```python
from build123d import *

# Parameters (mm, degrees)
BOSS_EXTRUDE1_DEPTH = 6.35
SKETCH3_R           = 3.96875
CUT_EXTRUDE1_DEPTH  = 7.35
SKETCH5_W           = 6.35
SKETCH5_H           = 12.7
CUT_EXTRUDE3_DEPTH  = 7.35
LPATTERN1_COUNT     = 16
LPATTERN1_PITCH     = 25.4
SKETCH6_W           = 6.35
SKETCH6_H           = 12.7
CUT_EXTRUDE4_DEPTH  = 7.35
LPATTERN2_COUNT     = 11
LPATTERN2_PITCH     = 25.4
SKETCH7_W           = 6.35
SKETCH7_H           = 12.7
SKETCH7_W_2         = 12.7
SKETCH7_H_2         = 6.35
CUT_EXTRUDE5_DEPTH  = 7.35
CUT_EXTRUDE6_DEPTH  = 7.35
LPATTERN3_COUNT     = 10
LPATTERN3_PITCH     = 25.4
SKETCH9_W           = 12.7
SKETCH9_H           = 6.35
CUT_EXTRUDE7_DEPTH  = 7.35
LPATTERN4_COUNT     = 8
LPATTERN4_PITCH     = 25.4
SKETCH10_R          = 3.175
CUT_EXTRUDE8_DEPTH  = 7.35
SKETCH11_R          = 3.96875
CUT_EXTRUDE9_DEPTH  = 7.35
SKETCH12_W          = 6.35
SKETCH12_H          = 12.7
CUT_EXTRUDE13_DEPTH = 7.35
CUT_EXTRUDE15_DEPTH = 7.35
CUT_EXTRUDE16_DEPTH = 7.35
SKETCH17_W          = 12.7
SKETCH17_H          = 6.35
CUT_EXTRUDE17_DEPTH = 7.35
LPATTERN5_COUNT     = 17
LPATTERN5_PITCH     = 25.4
LPATTERN6_COUNT     = 2
LPATTERN6_PITCH     = 120.65
SKETCH18_W          = 12.7
SKETCH18_H          = 6.35
CUT_EXTRUDE18_DEPTH = 7.35
LPATTERN7_COUNT     = 5
LPATTERN7_PITCH     = 25.4
CUT_EXTRUDE19_DEPTH = 7.35
SKETCH20_W          = 101.6
SKETCH20_H          = 57.15
CUT_EXTRUDE20_DEPTH = 7.35
CUT_EXTRUDE21_DEPTH = 7.35
CUT_EXTRUDE22_DEPTH = 7.35
BOSS_EXTRUDE4_DEPTH = 6.35
BOSS_EXTRUDE5_DEPTH = 6.35
SKETCH29_R          = 2.54
CUT_EXTRUDE23_DEPTH = 7.35
SKETCH30_R          = 1.75
CUT_EXTRUDE24_DEPTH = 7.35
SKETCH31_R          = 1.75
CUT_EXTRUDE25_DEPTH = 7.35
FILLET2_R           = 6.35


with BuildPart() as part:
    # Sketch2 → Boss-Extrude1 (new body)
    with BuildSketch(Plane(origin=(0, 0, 0), x_dir=(0, 0, -1), z_dir=(1, 0, 0))):
        Polygon((0, 0), (0, 294.450076882), (215.9, 419.1), (431.8, 419.1), (431.8, 0), (241.3, 0), (241.3, 38.1), (127, 38.1), (127, 0), align=None)
    extrude(amount=BOSS_EXTRUDE1_DEPTH)

    # Sketch3 → Cut-Extrude1 (cut, through all)
    with BuildSketch(Plane(origin=(6.35, 0, 0), x_dir=(0, 0, -1), z_dir=(1, 0, 0))):
        with Locations((63.5, 38.1)):
            Circle(SKETCH3_R)
        with Locations((368.3, 38.1)):
            Circle(SKETCH3_R)
    extrude(amount=-CUT_EXTRUDE1_DEPTH, mode=Mode.SUBTRACT)

    # Sketch5 → Cut-Extrude3 (cut, through all)
    with BuildSketch(Plane(origin=(6.35, 0, 0), x_dir=(0, 0, -1), z_dir=(1, 0, 0))):
        with Locations((428.625, 19.05)):
            Rectangle(SKETCH5_W, SKETCH5_H)
    cut_extrude3 = extrude(amount=-CUT_EXTRUDE3_DEPTH, mode=Mode.SUBTRACT)

    # LPattern1: Cut-Extrude3 ×16
    with Locations(*[(0, i * LPATTERN1_PITCH, 0) for i in range(1, LPATTERN1_COUNT)]):
        add(cut_extrude3, mode=Mode.SUBTRACT)

    # Sketch6 → Cut-Extrude4 (cut, through all)
    with BuildSketch(Plane(origin=(6.35, 0, 0), x_dir=(0, 0, -1), z_dir=(1, 0, 0))):
        with Locations((3.175, 19.05)):
            Rectangle(SKETCH6_W, SKETCH6_H)
    cut_extrude4 = extrude(amount=-CUT_EXTRUDE4_DEPTH, mode=Mode.SUBTRACT)

    # LPattern2: Cut-Extrude4 ×11
    with Locations(*[(0, i * LPATTERN2_PITCH, 0) for i in range(1, LPATTERN2_COUNT)]):
        add(cut_extrude4, mode=Mode.SUBTRACT)

    # Sketch7 → Cut-Extrude5 (cut, through all)
    with BuildSketch(Plane(origin=(6.35, 0, 0), x_dir=(0, 0, -1), z_dir=(1, 0, 0))):
        with Locations((123.825, 19.05)):
            Rectangle(SKETCH7_W, SKETCH7_H)
        with Locations((133.35, 41.275)):
            Rectangle(SKETCH7_W_2, SKETCH7_H_2)
        with Locations((158.75, 41.275)):
            Rectangle(SKETCH7_W_2, SKETCH7_H_2)
        with Locations((184.15, 41.275)):
            Rectangle(SKETCH7_W_2, SKETCH7_H_2)
        with Locations((244.475, 19.05)):
            Rectangle(SKETCH7_W, SKETCH7_H)
        with Locations((209.55, 41.275)):
            Rectangle(SKETCH7_W_2, SKETCH7_H_2)
        with Locations((234.95, 41.275)):
            Rectangle(SKETCH7_W_2, SKETCH7_H_2)
    extrude(amount=-CUT_EXTRUDE5_DEPTH, mode=Mode.SUBTRACT)

    # Sketch8 → Cut-Extrude6 (cut, through all)
    with BuildSketch(Plane(origin=(6.35, 0, 0), x_dir=(0, 0, -1), z_dir=(1, 0, 0))):
        Polygon((201.93507044, 411.037344159), (212.933593068, 417.387344159), (216.108593068, 411.888082845), (205.11007044, 405.538082845), align=None)
    cut_extrude6 = extrude(amount=-CUT_EXTRUDE6_DEPTH, mode=Mode.SUBTRACT)

    # LPattern3: Cut-Extrude6 ×10
    with Locations(*[Vector(0, -0.5, 0.866025404) * (i * LPATTERN3_PITCH) for i in range(1, LPATTERN3_COUNT)]):
        add(cut_extrude6, mode=Mode.SUBTRACT)

    # Sketch9 → Cut-Extrude7 (cut, through all)
    with BuildSketch(Plane(origin=(6.35, 0, 0), x_dir=(0, 0, -1), z_dir=(1, 0, 0))):
        with Locations((412.75, 415.925)):
            Rectangle(SKETCH9_W, SKETCH9_H)
    cut_extrude7 = extrude(amount=-CUT_EXTRUDE7_DEPTH, mode=Mode.SUBTRACT)

    # LPattern4: Cut-Extrude7 ×8
    with Locations(*[(0, 0, i * LPATTERN4_PITCH) for i in range(1, LPATTERN4_COUNT)]):
        add(cut_extrude7, mode=Mode.SUBTRACT)

    # Sketch10 → Cut-Extrude8 (cut, through all)
    with BuildSketch(Plane(origin=(6.35, 0, 0), x_dir=(0, 0, -1), z_dir=(1, 0, 0))):
        with Locations((222.25, 273.05)):
            Circle(SKETCH10_R)
        with Locations((222.25, 57.15)):
            Circle(SKETCH10_R)
        with Locations((146.05, 57.15)):
            Circle(SKETCH10_R)
        with Locations((146.05, 273.05)):
            Circle(SKETCH10_R)
    extrude(amount=-CUT_EXTRUDE8_DEPTH, mode=Mode.SUBTRACT)

    # Sketch11 → Cut-Extrude9 (cut, through all)
    with BuildSketch(Plane(origin=(6.35, 0, 0), x_dir=(0, 0, -1), z_dir=(1, 0, 0))):
        with Locations((38.1, 260.35)):
            Circle(SKETCH11_R)
        with Locations((266.7, 260.35)):
            Circle(SKETCH11_R)
    extrude(amount=-CUT_EXTRUDE9_DEPTH, mode=Mode.SUBTRACT)

    # Sketch12 → Cut-Extrude13 (cut, through all)
    with BuildSketch(Plane(origin=(6.35, 0, 0), x_dir=(0, 0, -1), z_dir=(1, 0, 0))):
        with Locations((123.825, 44.45)):
            Rectangle(SKETCH12_W, SKETCH12_H)
        with Locations((123.825, 69.85)):
            Rectangle(SKETCH12_W, SKETCH12_H)
        with Locations((123.825, 95.25)):
            Rectangle(SKETCH12_W, SKETCH12_H)
        with Locations((123.825, 120.65)):
            Rectangle(SKETCH12_W, SKETCH12_H)
    cut_extrude13 = extrude(amount=-CUT_EXTRUDE13_DEPTH, mode=Mode.SUBTRACT)

    # Sketch14 → Cut-Extrude15 (cut, through all)
    with BuildSketch(Plane(origin=(6.35, 0, 0), x_dir=(0, 0, -1), z_dir=(1, 0, 0))):
        Polygon((36.957231019, 315.787344159), (47.955753647, 322.137344159), (51.130753647, 316.638082845), (40.132231019, 310.288082845), align=None)
        Polygon((80.951321531, 341.187344159), (91.949844159, 347.537344159), (95.124844159, 342.038082845), (84.126321531, 335.688082845), align=None)
    extrude(amount=-CUT_EXTRUDE15_DEPTH, mode=Mode.SUBTRACT)

    # Sketch15 → Cut-Extrude16 (cut, through all)
    with BuildSketch(Plane(origin=(6.35, 0, 0), x_dir=(0, 0, -1), z_dir=(1, 0, 0))):
        with BuildLine():
            Line((62.129276275, 322.988082845), (31.558579521, 305.338082845))
            ThreePointArc((31.558579521, 305.338082845), (51.535904978, 302.314952438), (62.501260575, 319.285333297))
            ThreePointArc((62.501260575, 319.285333297), (62.408031035, 321.146027155), (62.129276275, 322.988082845))
        make_face()
        with BuildLine():
            Line((103.698495657, 346.988082845), (73.127798903, 329.338082845))
            ThreePointArc((73.127798903, 329.338082845), (93.10512436, 326.314952438), (104.070479957, 343.285333297))
            ThreePointArc((104.070479957, 343.285333297), (103.977250417, 345.146027155), (103.698495657, 346.988082845))
        make_face()
    extrude(amount=-CUT_EXTRUDE16_DEPTH, mode=Mode.SUBTRACT)

    # Sketch17 → Cut-Extrude17 (cut, through all)
    with BuildSketch(Plane(origin=(6.35, 0, 0), x_dir=(0, 0, -1), z_dir=(1, 0, 0))):
        with Locations((25.4, 142.875)):
            Rectangle(SKETCH17_W, SKETCH17_H)
    cut_extrude17 = extrude(amount=-CUT_EXTRUDE17_DEPTH, mode=Mode.SUBTRACT)

    # LPattern5: Cut-Extrude17 ×17
    with Locations(*[(0, 0, -i * LPATTERN5_PITCH) for i in range(1, LPATTERN5_COUNT)]):
        add(cut_extrude17, mode=Mode.SUBTRACT)

    # LPattern6: Cut-Extrude13 ×2
    with Locations(*[(0, 0, -i * LPATTERN6_PITCH) for i in range(1, LPATTERN6_COUNT)]):
        add(cut_extrude13, mode=Mode.SUBTRACT)

    # Sketch18 → Cut-Extrude18 (cut, through all)
    with BuildSketch(Plane(origin=(6.35, 0, 0), x_dir=(0, 0, -1), z_dir=(1, 0, 0))):
        with Locations((133.35, 117.475)):
            Rectangle(SKETCH18_W, SKETCH18_H)
    cut_extrude18 = extrude(amount=-CUT_EXTRUDE18_DEPTH, mode=Mode.SUBTRACT)

    # LPattern7: Cut-Extrude18 ×5
    with Locations(*[(0, 0, -i * LPATTERN7_PITCH) for i in range(1, LPATTERN7_COUNT)]):
        add(cut_extrude18, mode=Mode.SUBTRACT)

    # Sketch19 → Cut-Extrude19 (cut, through all)
    with BuildSketch(Plane(origin=(6.35, 0, 0), x_dir=(0, 0, -1), z_dir=(1, 0, 0))):
        Polygon((25.4, 279.785380045), (222.705909488, 393.7), (406.4, 393.7), (406.4, 165.1), (25.4, 165.1), align=None)
    extrude(amount=-CUT_EXTRUDE19_DEPTH, mode=Mode.SUBTRACT)

    # Sketch20 → Cut-Extrude20 (cut, through all)
    with BuildSketch(Plane(origin=(6.35, 0, 0), x_dir=(0, 0, -1), z_dir=(1, 0, 0))):
        with Locations((184.15, 79.375)):
            Rectangle(SKETCH20_W, SKETCH20_H)
    extrude(amount=-CUT_EXTRUDE20_DEPTH, mode=Mode.SUBTRACT)

    # Sketch21 → Cut-Extrude21 (cut, through all)
    with BuildSketch(Plane(origin=(6.35, 0, 0), x_dir=(0, 0, -1), z_dir=(1, 0, 0))):
        Polygon((266.7, 25.4), (308.202954744, 25.4), (406.4, 82.094090512), (406.4, 133.35), (266.7, 133.35), align=None)
        Polygon((25.4, 133.35), (25.4, 82.094090512), (101.6, 38.1), (101.6, 133.35), align=None)
        Polygon((25.4, 38.1), (25.4, 25.4), (47.397045256, 25.4), align=None)
    extrude(amount=-CUT_EXTRUDE21_DEPTH, mode=Mode.SUBTRACT)

    # Sketch22 → Cut-Extrude22 (cut, through all)
    with BuildSketch(Plane(origin=(6.35, 0, 0), x_dir=(0, 0, -1), z_dir=(1, 0, 0))):
        Polygon((384.402954744, 25.4), (406.4, 38.1), (406.4, 25.4), align=None)
    extrude(amount=-CUT_EXTRUDE22_DEPTH, mode=Mode.SUBTRACT)

    # Sketch26 → Boss-Extrude4 (add, through all)
    with BuildSketch(Plane(origin=(6.35, 0, 0), x_dir=(0, 0, -1), z_dir=(1, 0, 0))):
        Polygon((266.7, 133.35), (266.7, 126.280871047), (278.944090512, 133.35), align=None)
        Polygon((89.355909488, 133.35), (101.6, 126.280871047), (101.6, 133.35), align=None)
        Polygon((266.7, 32.469128953), (278.944090512, 25.4), (266.7, 25.4), align=None)
        Polygon((133.35, 107.95), (133.35, 100.880871047), (145.594090512, 107.95), align=None)
        Polygon((234.95, 107.95), (222.705909488, 107.95), (234.95, 100.880871047), align=None)
        Polygon((133.35, 50.8), (145.594090512, 50.8), (133.35, 57.869128953), align=None)
        Polygon((234.95, 50.8), (222.705909488, 50.8), (234.95, 57.869128953), align=None)
    extrude(amount=-BOSS_EXTRUDE4_DEPTH)


with BuildPart() as body_2:
    # Sketch27 → Boss-Extrude5 (new body)
    with BuildSketch(Plane(origin=(6.35, 0, 0), x_dir=(0, 0, -1), z_dir=(1, 0, 0))):
        Polygon((12.7, 163.83), (12.7, 12.7), (114.3, 12.7), (114.3, 50.8), (254, 50.8), (254, 12.7), (419.1, 12.7), (419.1, 163.83), align=None)
    extrude(amount=-BOSS_EXTRUDE5_DEPTH)

    # Sketch29 → Cut-Extrude23 (cut, through all)
    with BuildSketch(Plane(origin=(6.35, 0, 0), x_dir=(0, 0, -1), z_dir=(1, 0, 0))):
        with Locations((38.1, 157.1625)):
            Circle(SKETCH29_R)
        with Locations((88.9, 157.1625)):
            Circle(SKETCH29_R)
        with Locations((139.7, 157.1625)):
            Circle(SKETCH29_R)
        with Locations((190.5, 157.1625)):
            Circle(SKETCH29_R)
        with Locations((241.3, 157.1625)):
            Circle(SKETCH29_R)
        with Locations((292.1, 157.1625)):
            Circle(SKETCH29_R)
        with Locations((342.9, 157.1625)):
            Circle(SKETCH29_R)
        with Locations((393.7, 157.1625)):
            Circle(SKETCH29_R)
    extrude(amount=-CUT_EXTRUDE23_DEPTH, mode=Mode.SUBTRACT)

    # Sketch30 → Cut-Extrude24 (cut, through all)
    with BuildSketch(Plane(origin=(6.35, 0, 0), x_dir=(0, 0, -1), z_dir=(1, 0, 0))):
        with Locations((22.225, 58.42)):
            Circle(SKETCH30_R)
        with Locations((104.775, 22.225)):
            Circle(SKETCH30_R)
        with Locations((263.525, 22.225)):
            Circle(SKETCH30_R)
        with Locations((409.575, 58.42)):
            Circle(SKETCH30_R)
    extrude(amount=-CUT_EXTRUDE24_DEPTH, mode=Mode.SUBTRACT)

    # Sketch31 → Cut-Extrude25 (cut, through all)
    with BuildSketch(Plane(origin=(6.35, 0, 0), x_dir=(0, 0, -1), z_dir=(1, 0, 0))):
        with Locations((260.35, 133.35)):
            Circle(SKETCH31_R)
        with Locations((409.575, 133.35)):
            Circle(SKETCH31_R)
    extrude(amount=-CUT_EXTRUDE25_DEPTH, mode=Mode.SUBTRACT)

    # Fillet2
    fillet2_edges = [body_2.edges().sort_by_distance(p)[0] for p in [
        (3.175, 163.83, -419.1),
        (3.175, 12.7, -419.1),
        (3.175, 12.7, -254),
        (3.175, 50.8, -254),
        (3.175, 50.8, -114.3),
        (3.175, 12.7, -114.3),
        (3.175, 12.7, -12.7),
        (3.175, 163.83, -12.7),
    ]]
    fillet(fillet2_edges, radius=FILLET2_R)


solid = body_2.part
```
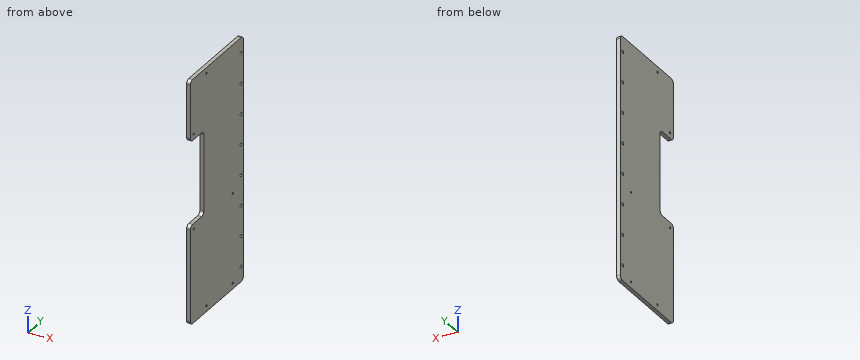
Build history of the part. All positions in model axes, mm. Round coordinates to 2 decimals unless told otherwise and drop trailing zeros. Write each loop counter-clockwise with the first axis right and the second up, starting at its lowest first coordinate (ties: lowest second). Pieces come first, ordered by that corner, then holes.
1) Pin check, flat tip, straight feed: pin 1 (3 mm diameter, centred on x = 3, z = -206, fed in from -Y). Stop position of the tip, or through.
2) Drill centre lines: probe 1 along Z at (x, y) = (5.25, 133.35) (3 decimals); probe 2 along Z at (x, y) = (4.5, 21); probe 3 along Y at (x, z) = (2, -260.35). Where is each one in solid material? Low to high.
3) Band-saw the part on A-A, the plane x = 1. Give the number of separate pieces and of enclosed holes in the cut face, and give its area (3 significant figures).
4) Band-saw the part on B-B, the plane z = -149.5. List the corners of the cut face in (x, y).
Ans:
1. pin 1: stops at y = 50.8
2. probe 1: z = -419.1 to -411.325, -407.825 to -262.1, -258.6 to -12.7
2. probe 2: z = -419.1 to -264.77, -262.28 to -254, -114.3 to -106.02, -103.53 to -12.7
2. probe 3: y = 12.7 to 131.6, 135.1 to 163.83
3. separate pieces: 1
3. enclosed holes: 14
3. area: 55,800 mm2
4. outline: (0, 50.8) - (6.35, 50.8) - (6.35, 163.83) - (0, 163.83) - close
